```python
from build123d import *

# Parameters (mm, degrees)
SKIZZE1_W                       = 44.5
SKIZZE1_H                       = 22.5
SKIZZE1_R                       = 1.65
AUFSATZ_LINEAR_AUSTRAGEN1_DEPTH = 5
VERRUNDUNG1_R                   = 2
SKIZZE2_R                       = 2.95
SCHNITT_LINEAR_AUSTRAGEN1_DEPTH = 3


with BuildPart() as part:
    # Skizze1 → Aufsatz-Linear austragen1 (new body)
    with BuildSketch(Plane.XY):
        Rectangle(SKIZZE1_W, SKIZZE1_H)
        with Locations((-18.6, 7.25)):
            Circle(SKIZZE1_R, mode=Mode.SUBTRACT)
        with Locations(Location((18.6, 7.25, 0), (0, 0, 180))):
            Circle(SKIZZE1_R, mode=Mode.SUBTRACT)
        with Locations((18.6, -7.25)):
            Circle(SKIZZE1_R, mode=Mode.SUBTRACT)
        with Locations(Location((-18.6, -7.25, 0), (0, 0, 180))):
            Circle(SKIZZE1_R, mode=Mode.SUBTRACT)
    extrude(amount=AUFSATZ_LINEAR_AUSTRAGEN1_DEPTH)

    # Verrundung1
    verrundung1_edges = [part.edges().sort_by_distance(p)[0] for p in [
        (-22.25, 0, 5),
        (0, -11.25, 5),
        (22.25, 0, 5),
        (0, 11.25, 5),
    ]]
    fillet(verrundung1_edges, radius=VERRUNDUNG1_R - 0.0001)  # a hair under: the kernel refuses the full size

    # Skizze2 → Schnitt-Linear austragen1 (cut)
    with BuildSketch(Plane.XY.offset(5)):
        with Locations(Location((-18.6, 7.25, 0), (0, 0, 42.684910775))):
            Circle(SKIZZE2_R)
        with Locations(Location((-18.6, -7.25, 0), (0, 0, 317.315089225))):
            Circle(SKIZZE2_R)
        with Locations(Location((18.6, -7.25, 0), (0, 0, 310.187569286))):
            Circle(SKIZZE2_R)
        with Locations(Location((18.6, 7.25, 0), (0, 0, 49.812430991))):
            Circle(SKIZZE2_R)
    extrude(amount=-SCHNITT_LINEAR_AUSTRAGEN1_DEPTH, mode=Mode.SUBTRACT)


solid = part.part
```
Model file for the job. Use its own axes, mm. A direction names the side the tool comes from. Round coordinates to 2 decimals unless told otherwise and drop trailing zeros. Write each loop counter-clockwise with the first axis right and the second up, starting at its lowest first coordinate (ties: lowest second). Pieces come first, ordered by that corner, then holes. Notation, with made-up numbers: (63, -3.5) - (95, -3.5) arc R19 cw to (95, 20.5) - close; hole circle Ø3 at (-24.5, 43). An arc over 180 degrees is marked (long way). Use CSV: the item, a comma, the result in double quotes. Start each with the question number.
Item 1: Drill centre lines: L1, parallel to X at y = -7.25, z = 1.4; L2, parallel to Y at x = -18.6, z = 1.6; L3, parallel to X at y = 5, z = 4.6. Where is each one in solid material? Low to high. Write a range as [from, to].
Item 2: Pin check, flat tips, straight feed: P1, Ø1, axis at y = 3.5, z = 4.5, coming from the -X side; P2, Ø4, axis at x = 18.6, y = -7.25, coming from the -Z side; P3, Ø3, axis at x = -19, y = -7.5, coming from the +Z side. Stop position of each tip, or through.
Item 3: Band-saw the part on A-A (z = 1.35). Write the cut outline in (x, y), and give its area (3 significant figures).
Item 4: Two-plate mould, pull along Y, no slides. Class faces 3 (the face through (0, -11.25, 1)), 4 (the face through (-16.8, 7.2, 2)), 5 (the face through (0.31, 10.68, 4.4)), 6 (the face through (-17.076, 6.618, 0.986)): released by +Y, released by -Y, zero draft, split by the parting line, or undercut.
Item 5: Band-saw the part on C-C (y = -7.75). Write the cut outline in (x, z), and give its area (3 significant figures).
Item 6: Band-saw the part on B-B (x = -18.6). Write the cut outline in (y, z).
Item 7: Tool access for faces 1 (the face through (16.95, -7.18, 0.99)), 2 (the face through (16.797, -4.915, 3.521)): list every direction of +Z, -Z, +X, -X, +Y, -Y with a clear straight run to the whole face (end or side of a thin tool).
Item 8: Band-saw the part on D-D (x = 5.5). Write the cut outline in (y, z).
Checked values:
1,L1,"x = [-22.25, -20.25], [-16.95, 16.95], [20.25, 22.25]"
1,L2,"y = [-11.25, -8.9], [-5.6, 5.6], [8.9, 11.25]"
1,L3,"x = [-21.45, -20.51], [-16.69, 16.69], [20.51, 21.45]"
2,P1,"stops at x = -21.98"
2,P2,"stops at z = 0"
2,P3,"stops at z = 2"
3,outline,"(-22.25, -11.25) - (22.25, -11.25) - (22.25, 11.25) - (-22.25, 11.25) - close; hole circle Ø3.3 at (-18.6, -7.25); hole circle Ø3.3 at (-18.6, 7.25); hole circle Ø3.3 at (18.6, -7.25); hole circle Ø3.3 at (18.6, 7.25)"
3,area,"967 mm²"
4,face 3,"released by -Y"
4,face 4,"undercut"
4,face 5,"released by +Y"
4,face 6,"undercut"
5,outline,"(-22.25, 0) - (-20.17, 0) - (-20.17, 2) - (-21.51, 2) - (-21.51, 4.56) arc R2 ccw to (-22.25, 3) - close; (-17.03, 0) - (17.03, 0) - (17.03, 2) - (15.69, 2) - (15.69, 5) - (-15.69, 5) - (-15.69, 2) - (-17.03, 2) - close; (20.17, 0) - (22.25, 0) - (22.25, 3) arc R2 ccw to (21.51, 4.56) - (21.51, 2) - (20.17, 2) - close"
5,area,"174 mm²"
6,outline,"(-11.25, 0) - (-8.9, 0) - (-8.9, 2) - (-10.2, 2) - (-10.2, 4.76) arc R2 ccw to (-11.25, 3) - close; (-5.6, 0) - (5.6, 0) - (5.6, 2) - (4.3, 2) - (4.3, 5) - (-4.3, 5) - (-4.3, 2) - (-5.6, 2) - close; (8.9, 0) - (11.25, 0) - (11.25, 3) arc R2 ccw to (10.2, 4.76) - (10.2, 2) - (8.9, 2) - close"
7,face 1,"+Z, -Z"
7,face 2,"+Z"
8,outline,"(-11.25, 0) - (11.25, 0) - (11.25, 3) arc R2 ccw to (9.25, 5) - (-9.25, 5) arc R2 ccw to (-11.25, 3) - close"
